Here's the drawing with two shaded views (mm, measured from the low corner). I have some questions. A direction names the side the tool comes from. Give positions to 0.01 mm unless a question says otherwise; leave off trailing zeros. Write each loop counter-clockwise with the first axis right and the second up, starting at its lowest first coordinate (ties: lowest second). Pieces come first, ordered by that corner, then holes.
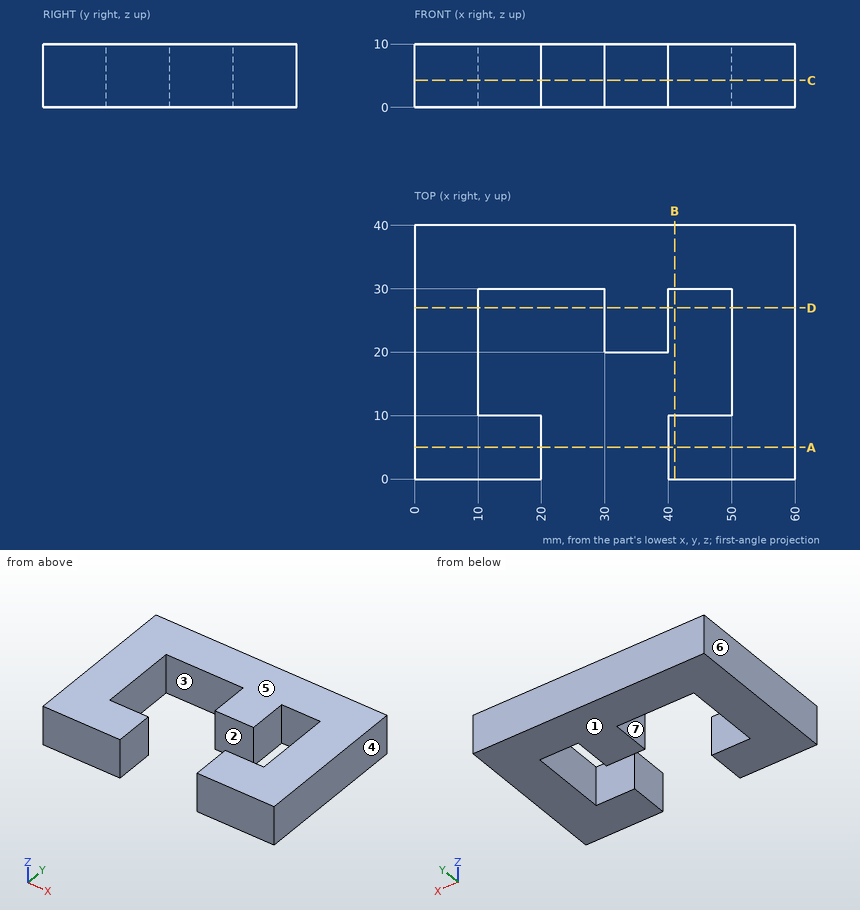
1) If we mould it in two halves opening along X, with no side actions, what happens to the marked faces 4, 5, 6 and 7? For each: +X half, -X half, draft (parallel to the pull), parting line (faces both ways), or undercut.
Values follow:
face 4: +X half
face 5: draft
face 6: -X half
face 7: undercut
2) Suppose I cut it at D-D on y = 27. Write out the boundary of the cut face in (x, z), plus the area to 3 significant figures.
Values follow:
outline: (0, 0) - (10, 0) - (10, 10) - (0, 10) - close; (30, 0) - (40, 0) - (40, 10) - (30, 10) - close; (50, 0) - (60, 0) - (60, 10) - (50, 10) - close
area: 300 mm2
3) Suppose I cut it at B-B on x = 41. Write out the boundary of the cut face in (y, z), plus the area to 3 significant figures.
Values follow:
outline: (0, 0) - (10, 0) - (10, 10) - (0, 10) - close; (30, 0) - (40, 0) - (40, 10) - (30, 10) - close
area: 200 mm2
4) Suppose I cut it at C-C on z = 4.25. Write out the boundary of the cut face in (x, y).
Values follow:
outline: (0, 0) - (20, 0) - (20, 10) - (10, 10) - (10, 30) - (30, 30) - (30, 20) - (40, 20) - (40, 30) - (50, 30) - (50, 10) - (40, 10) - (40, 0) - (60, 0) - (60, 40) - (0, 40) - close
5) Suppose I cut it at A-A on y = 5. Write out the boundary of the cut face in (x, z).
Values follow:
outline: (0, 0) - (20, 0) - (20, 10) - (0, 10) - close; (40, 0) - (60, 0) - (60, 10) - (40, 10) - close
6) Please list where these lines run through material, in increasing order: L1, parallel to X at y = 20.5, z = 2.5; L2, parallel to Y at x = 44, z = 8; L3, parallel to X at y = 7, z = 3.25.
Values follow:
L1: x = 0 to 10, 30 to 40, 50 to 60
L2: y = 0 to 10, 30 to 40
L3: x = 0 to 20, 40 to 60
7) For the marked faces 1, 2 and 3, which set-ups out of +Z, -Z, +X, -X, +Y, -Y let a thin tool reach every point of the face, with its end or its side?
Values follow:
face 1: -Z, +X, -X, +Y, -Y
face 2: +Z, -Z, -Y
face 3: +Z, -Z
